```python
from build123d import *

# Parameters (mm, degrees)
F1_DEPTH = 44.45
F2_DEPTH = 25.4


with BuildPart() as f1:
    # F0 (on Top) → F1 (new body)
    with BuildSketch(Plane.XY):
        with BuildLine():
            Line((-38.1, -12.7), (-38.1, -25.4))
            ThreePointArc((-38.1, -25.4), (-20.139488, -17.960512), (-12.7, 0))
            ThreePointArc((-12.7, 0), (-20.139488, 17.960512), (-38.1, 25.4))
            Line((-38.1, 25.4), (-38.1, 12.7))
            ThreePointArc((-38.1, 12.7), (-29.119744, 8.980256), (-25.4, 0))
            ThreePointArc((-25.4, 0), (-29.119744, -8.980256), (-38.1, -12.7))
        make_face()
        with BuildLine():
            ThreePointArc((-38.1, 25.4), (-63.5, 0), (-38.1, -25.4))
            Line((-38.1, -25.4), (-38.1, -12.7))
            ThreePointArc((-38.1, -12.7), (-50.8, 0), (-38.1, 12.7))
            Line((-38.1, 12.7), (-38.1, 25.4))
        make_face()
    extrude(amount=F1_DEPTH)

    # F0 (on Top) → F2 (join)
    with BuildSketch(Plane.XY):
        with BuildLine():
            ThreePointArc((-12.7, 0), (-20.139488, -17.960512), (-38.1, -25.4))
            Line((-38.1, -25.4), (38.1, -25.4))
            Line((38.1, -25.4), (38.1, -12.7))
            ThreePointArc((38.1, -12.7), (25.4, 0), (38.1, 12.7))
            Line((38.1, 12.7), (38.1, 25.4))
            Line((38.1, 25.4), (-38.1, 25.4))
            ThreePointArc((-38.1, 25.4), (-20.139488, 17.960512), (-12.7, 0))
        make_face()
        with BuildLine():
            ThreePointArc((-38.1, 25.4), (-63.5, 0), (-38.1, -25.4))
            Line((-38.1, -25.4), (-38.1, -12.7))
            ThreePointArc((-38.1, -12.7), (-50.8, 0), (-38.1, 12.7))
            Line((-38.1, 12.7), (-38.1, 25.4))
        make_face()
        with BuildLine():
            Line((38.1, -12.7), (38.1, -25.4))
            ThreePointArc((38.1, -25.4), (63.5, 0), (38.1, 25.4))
            Line((38.1, 25.4), (38.1, 12.7))
            ThreePointArc((38.1, 12.7), (47.080256, 8.980256), (50.8, 0))
            ThreePointArc((50.8, 0), (47.080256, -8.980256), (38.1, -12.7))
        make_face()
    extrude(amount=F2_DEPTH)


solid = f1.part
```
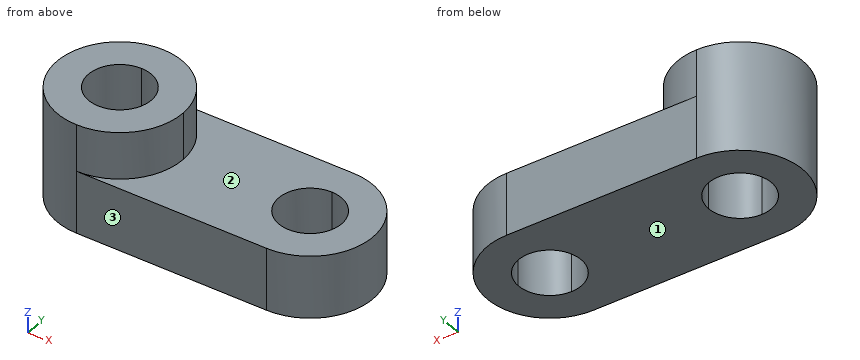
Part model, mm, in its own coordinate system. Face numbers are marked on the shaded views. Round coordinates to 2 decimals unless told otherwise and drop trailing zeros. Order: outer loops, then holes, each group sorted by start corner. A loop starts at its lowest first (then second) coordinate and runs counter-clockwise, first axis right, second up. Notation, with made-up numbers: M -36,64.5 L 2,64.5 A19 ccw 2,70.5 Z; hole C 69,75 d10. An arc over 180 degrees is marked long. Put each result on its own line as item: value. Start each with the question number.
1. Slice it at D-D on z = 27. List the corners of the cut face in (x, y), then the cut area to 3 significant figures.
2. Slice it at A-A on z = 4.5. List the corners of the cut face in (x, y).
3. Drill centre lines: probe 1 along X at (y, z) = (11.5, 3.5); probe 2 along X at (y, z) = (1.5, 14); probe 3 along Z at (x, y) = (4, 15.5). Where is each one in solid material? Low to high. Write a range as [from, to].
4. Slice it at B-B on y = -9. List the corners of the cut face in (x, z).
5. Drop flat-ended pins along their axis: pin 1 (1 mm diameter, centred on y = -18.5, z = 34, fed in from +X); pin 2 (15 mm diameter, centred on x = 37.5, y = 11, fed in from +Z); pin 3 (12 mm diameter, centred on y = -6, z = 31.5, fed in from +X). Give the stop position or say it passes through.
6. Slice it at C-C on x = 44. List the corners of the cut face in (y, z).
7. Two-plate mould, pull along Z, no slides. Class the marked faces 1, 2 and 3: +Z half, -Z half, draft (parallel to the pull), parting line (faces both ways), or undercut.
Findings:
1. outline: M -38.1,-25.4 A25.4 ccw -12.7,0 A25.4 ccw long Z; hole C -38.1,0 d25.4
1. area: 1,520 mm2
2. outline: M -38.1,-25.4 L 38.1,-25.4 A25.4 ccw 38.1,25.4 L -38.1,25.4 A25.4 ccw Z; hole C -38.1,0 d25.4; hole C 38.1,0 d25.4
3. probe 1: [-60.75, -43.49], [-32.71, 32.71], [43.49, 60.75]
3. probe 2: [-63.46, -50.71], [-25.49, 25.49], [50.71, 63.46]
3. probe 3: [0, 25.4]
4. outline: M -61.85,0 L -47.06,0 L -47.06,44.45 L -61.85,44.45 Z; M -29.14,0 L 29.14,0 L 29.14,25.4 L -14.35,25.4 L -14.35,44.45 L -29.14,44.45 Z; M 47.06,0 L 61.85,0 L 61.85,25.4 L 47.06,25.4 Z
5. pin 1: x = -20.18
5. pin 2: z = 25.4
5. pin 3: x = -12.7
6. outline: M -24.71,0 L -11.25,0 L -11.25,25.4 L -24.71,25.4 Z; M 11.25,0 L 24.71,0 L 24.71,25.4 L 11.25,25.4 Z
7. face 1: -Z half
7. face 2: +Z half
7. face 3: draft
